```python
from build123d import *

# Parameters (mm, degrees)
SKETCH1_W           = 20
SKETCH1_H           = 20
BOSS_EXTRUDE1_DEPTH = 5
SKETCH3_W           = 4
SKETCH3_H           = 20
BOSS_EXTRUDE2_DEPTH = 10
SKETCH4_R           = 10
BOSS_EXTRUDE3_DEPTH = 4
BOSS_EXTRUDE4_START = -4
SKETCH5_R           = 10
BOSS_EXTRUDE4_DEPTH = 4
SKETCH6_R           = 1.1
CUT_EXTRUDE1_DEPTH  = 36.791060336
SKETCH7_R           = 0.5
CUT_EXTRUDE2_DEPTH  = 35.641016151
SKETCH9_R           = 6
BOSS_EXTRUDE5_DEPTH = 4
SKETCH10_R          = 1.1
CUT_EXTRUDE3_DEPTH  = 4
FILLET1_R           = 2


with BuildPart() as part:
    # Sketch1 → Boss-Extrude1 (new body)
    with BuildSketch(Plane(origin=(0, 0, 0), x_dir=(1, 0, 0), z_dir=(0, 1, 0))):
        with Locations((10, 10)):
            Rectangle(SKETCH1_W, SKETCH1_H)
    extrude(amount=BOSS_EXTRUDE1_DEPTH)

    # Sketch3 → Boss-Extrude2 (add)
    with BuildSketch(Plane(origin=(0, 5, 0), x_dir=(1, 0, 0), z_dir=(0, 1, 0))):
        with Locations((6, 10)):
            Rectangle(SKETCH3_W, SKETCH3_H)
        with Locations((14, 10)):
            Rectangle(SKETCH3_W, SKETCH3_H)
    extrude(amount=BOSS_EXTRUDE2_DEPTH)

    # Sketch4 → Boss-Extrude3 (add)
    with BuildSketch(Plane.ZY.offset(-4)):
        with Locations((-10, 15)):
            Circle(SKETCH4_R)
    extrude(amount=-BOSS_EXTRUDE3_DEPTH)

    # Sketch5 → Boss-Extrude4 (add)
    with BuildSketch(Plane(origin=(16, 0, 0), x_dir=(0, 0, -1), z_dir=(1, 0, 0)).offset(BOSS_EXTRUDE4_START)):
        with Locations((10, 15)):
            Circle(SKETCH5_R)
    extrude(amount=BOSS_EXTRUDE4_DEPTH)

    # Sketch6 → Cut-Extrude1 (cut, through all)
    with BuildSketch(Plane.ZY.offset(-4)):
        with Locations((-10, 15)):
            Circle(SKETCH6_R)
    extrude(amount=-CUT_EXTRUDE1_DEPTH, mode=Mode.SUBTRACT)

    # Sketch7 → Cut-Extrude2 (cut, through all)
    with BuildSketch(Plane(origin=(0, 5, 0), x_dir=(1, 0, 0), z_dir=(0, 1, 0))):
        with Locations(Location((10, 4, 0), (0, 0, 270))):
            Circle(SKETCH7_R)
        with Locations(Location((10, 16, 0), (0, 0, 90))):
            Circle(SKETCH7_R)
    extrude(amount=-CUT_EXTRUDE2_DEPTH, mode=Mode.SUBTRACT)

    # Sketch9 → Boss-Extrude5 (add)
    with BuildSketch(Plane(origin=(8, 0, 0), x_dir=(0, 0, -1), z_dir=(1, 0, 0))):
        with Locations(Location((10, 15, 0), (0, 0, 180))):
            Circle(SKETCH9_R)
    extrude(amount=BOSS_EXTRUDE5_DEPTH)

    # Sketch10 → Cut-Extrude3 (cut)
    with BuildSketch(Plane(origin=(8, 0, 0), x_dir=(0, 0, -1), z_dir=(1, 0, 0))):
        with Locations(Location((10, 15, 0), (0, 0, 180))):
            Circle(SKETCH10_R)
    extrude(amount=CUT_EXTRUDE3_DEPTH, mode=Mode.SUBTRACT)

    # Fillet1
    fillet1_edges = [part.edges().sort_by_distance(p)[0] for p in [
        (12, 15, -16),
        (8, 15, -16),
    ]]
    fillet(fillet1_edges, radius=FILLET1_R - 0.0001)  # a hair under: the kernel refuses the full size


solid = part.part
```
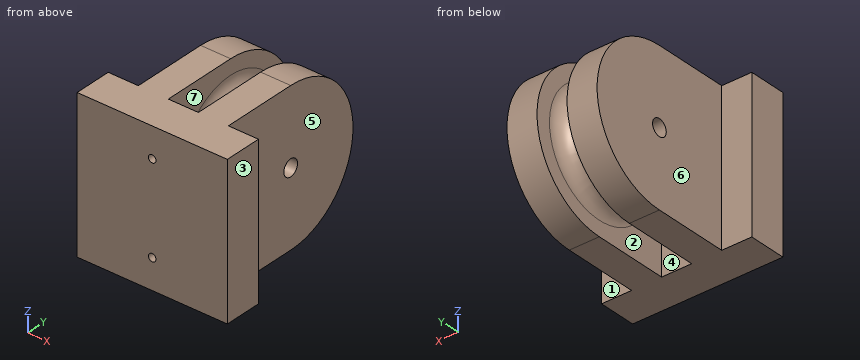
For this review, take the finished solid that the model builds, in its own axes (mm). Face numbers are marked on the shaded views. A direction names the side the tool comes from. Round coordinates to 2 decimals unless told otherwise and drop trailing zeros. Write each loop counter-clockwise with the first axis right and the second up, starting at its lowest first coordinate (ties: lowest second). Pieces come first, ordered by that corner, then holes. Notation, with made-up numbers: (27.25, 57) -> (60.25, 57) arc R26 ccw to (60.25, 93) -> close; hole circle Ø3 at (79.5, 83). An arc over 180 degrees is marked (long way). Use one line per item in the form item = value.
1) To check wall thickness, follow L1, parallel to X at y = 6.5, z = -5.5; L2, parallel to Y at x = 13.35, z = -10; L3, parallel to X at y = 1, z = -4. State the ranges of each line that lie inside material, in increasing order. Write a range as from..to.
Found:
L1 = 4..8, 12..16
L2 = 0..13.9, 16.1..25
L3 = 0..9.5, 10.5..20
2) Tool access review of the marked faces 5, 6 and 7: name each direction out of +Z, -Z, +X, -X, +Y, -Y from which nothing blocks a thin tool from reaching the whole face with its end or side.
Found:
face_5 = +Z, -Z, +X, +Y
face_6 = +Z, -Z, -X, +Y
face_7 = none
3) Take a section at A-A, the plane z = -10. Count the separate pieces of the cut face and the enclosed holes in it, and give its area (3 significant figures).
Found:
separate_pieces = 2
enclosed_holes = 1
area = 285 mm2
4) Take a section at B-B, the plane x = 15.25. Write out the cut boundary in (y, z), and give its area (3 significant figures).
Found:
outline = (0, -20) -> (15, -20) arc R10 ccw to (15, 0) -> (0, 0) -> close; hole circle Ø2.2 at (15, -10)
area = 453 mm2
5) Take a section at C-C, the plane x = 18.75. Write out the cut boundary in (y, z).
Found:
outline = (0, -20) -> (5, -20) -> (5, 0) -> (0, 0) -> close
6) Mouldability with a two-part tool opening along X and no side actions: class the marked faces 1, 2, 3 and 4 as +X half, -X half, draft (parallel to the pull), parting line (faces both ways), or undercut.
Found:
face_1 = draft
face_2 = undercut
face_3 = +X half
face_4 = undercut
7) Clearance check with flat-ended pins moving along their axes: pin 1 (3 mm diameter, centred on y = 18.5, z = -15, fed in from +X); pin 2 (6 mm diameter, centred on y = 14, z = -9, fed in from -X); pin 3 (1.2 mm diameter, centred on x = 3, z = -15, fed in from +Y). State where each tip first meets the part, or that it passes through.
Found:
pin_1 = 16
pin_2 = 4
pin_3 = 5
